Autodesk Inventor part; units mm, degrees
ref_plane "YZ Plane" through (0, 0, 0) normal (1, 0, 0) x (0, 1, 0)
ref_plane "XZ Plane" through (0, 0, 0) normal (0, 1, 0) x (-1, 0, 0)
ref_plane "XY Plane" through (0, 0, 0) normal (0, 0, 1) x (1, 0, 0)
sketch "Szkic1" plane through (0, 0, 0) normal (0, 1, 0) x (-1, 0, 0)
  line L0 (0, 0) -> (150, 0)
  line L1 (150, 0) -> (150, -5)
  line L2 (150, -5) -> (0, -5)
  line L3 (0, -5) -> (0, 0)
  dimension "d0" = 150
  dimension "d1" = 5
extrude "Wyciągnięcie proste1" add sketch "Szkic1" along normal blind 20
sketch "Szkic2" plane through (0, 0, -5) normal (0, 0, -1) x (-1, 0, 0)
  line L0 (0, 0) -> (0, 20)
  circle A0 centre (0, 10) radius 2.95
  line L1 (0, 20) -> (-2, 20)
  line L2 (0, 0) -> (-2, 0)
  arc A1 (-2, 20) -> (-2, 0) centre (9.1803, 10) ccw
  line L3 (0, 10) -> (150, 10)
  line L4 (150, 10) -> (138.5, 10)
  line L5 (138.5, 10) -> (170.9, 10)
  line L6 (150, 0) -> (150, 20)
  line L7 (138.5, 10) -> (170.9, 10) construction
  line L8 (138.5, 10) -> (170.9, 10)
  line L9 (170.9, 10) -> (170.9, 16.16)
  line L10 (170.9, 16.16) -> (138.5, 16.16)
  line L11 (138.5, 16.16) -> (138.5, 10)
  line L12 (138.5, 10) -> (170.9, 10)
  line L13 (170.9, 10) -> (170.9, 3.84)
  line L14 (170.9, 3.84) -> (138.5, 3.84)
  line L15 (138.5, 3.84) -> (138.5, 10)
  line L16 (0, 0) -> (150, 0)
  line L17 (0, 20) -> (150, 20)
  arc A2 (138.5, 0) -> (138.5, 20) centre (154.9429, 10) ccw
  point P0 (150, 3.84)
  point P1 (150, 16.16)
  point P2 (0, 7.05)
  point P3 (0, 12.95)
  dimension "d4" = 5.9
  dimension "d5" = 2
  dimension "d6" = 2
  dimension "d7" = 15
  dimension "d8" = 150
  dimension "d9" = 11.5
  dimension "d10" = 32.4
  dimension "d11" = 0
  dimension "d12" = 6.16
  dimension "d13" = 6.16
extrude "Wyciągnięcie proste2" add sketch "Szkic2" against normal blind 5 contours L2 A1 L1 L0 A0 | L16 L6 L14 L13 L9 L10 L17 A2
sketch "Szkic3" plane through (2, 20, -5) normal (0, 0, -1) x (-1, 0, 0)
  arc A0 (2, -7.05) -> (2, -12.95) centre (2, -10) ccw
  circle A1 centre (2, -10) radius 2.95
  line L0 (152, -16.16) -> (152, -3.84)
  line L1 (152, -16.16) -> (150.5, -16.16)
  line L2 (150.5, -16.16) -> (150.5, -3.84)
  line L3 (150.5, -3.84) -> (152, -3.84)
  line L4 (140.5, -16.16) -> (10.5, -16.16)
  line L5 (10.5, -16.16) -> (10.5, -3.84)
  line L6 (10.5, -3.84) -> (140.5, -3.84)
  line L7 (140.5, -3.84) -> (140.5, -16.16)
  line L8 (150.5, -16.16) -> (150.3, -16.16)
  line L9 (150.3, -16.16) -> (150.3, -3.84)
  line L10 (150.3, -3.84) -> (150.5, -3.84)
  line L11 (152, -16.16) -> (140.5, -16.16)
  line L12 (140.5, -16.16) -> (140.5, -3.84)
  line L13 (140.5, -3.84) -> (152, -3.84)
  line L14 (152, -3.84) -> (152, -16.16)
  point P0 (2, -20)
  dimension "d16" = 1.5
  dimension "d17" = 130
  dimension "d18" = 12.32
  dimension "d21" = 0.2
  dimension "d24" = 11.5
extrude "Wyciągnięcie proste3" cut sketch "Szkic3" against normal through all
sketch "Szkic5" plane through (2, 20, -5) normal (0, 0, -1) x (-1, 0, 0)
  circle A0 centre (2, -10) radius 2.95
  line L0 (2, -10) -> (152, -10)
  line L1 (2, -10) -> (152, -10) construction
  circle A1 centre (152, -10) radius 5.0551
  line L2 (152, -10) -> (145.8, -10)
  line L3 (145.8, -10) -> (145.8, -3.84)
  line L4 (10.5, -3.84) -> (172.9, -3.84)
  line L5 (145.8, -3.84) -> (140.8, -3.84)
  line L6 (140.8, -3.84) -> (140.8, -16.16)
  line L7 (172.9, -16.16) -> (10.5, -16.16)
  line L8 (145.8, -10) -> (145.8, -16.16)
  line L9 (145.8, -16.16) -> (140.8, -16.16)
  line L10 (10.5, -16.16) -> (10.5, -3.84)
  line L11 (10.5, -16.16) -> (44.3489, -3.84)
  line L12 (10.5, -16.16) -> (46.5213, -16.16) construction
  line L13 (44.3489, -3.84) -> (54.3489, -3.84)
  line L14 (10.5, -16.16) -> (20.5, -16.16)
  line L15 (20.5, -16.16) -> (54.3489, -3.84)
  line L16 (20.5, -16.16) -> (30.5, -16.16)
  line L17 (54.3489, -3.84) -> (64.3489, -3.84)
  line L18 (64.3489, -3.84) -> (30.5, -16.16)
  line L19 (44.3489, -3.84) -> (34.3489, -3.84)
  line L20 (10.5, -16.16) -> (0.5, -16.16)
  line L21 (0.5, -16.16) -> (34.3489, -3.84)
  line L22 (40.5, -16.16) -> (74.3489, -3.84)
  line L23 (50.5, -16.16) -> (84.3489, -3.84)
  line L24 (94.3489, -3.84) -> (60.5, -16.16)
  line L25 (30.5, -16.16) -> (64.3489, -3.84)
  line L26 (70.5, -16.16) -> (104.3489, -3.84)
  line L27 (80.5, -16.16) -> (114.3489, -3.84)
  line L28 (124.3489, -3.84) -> (90.5, -16.16)
  line L29 (60.5, -16.16) -> (94.3489, -3.84)
  line L30 (100.5, -16.16) -> (134.3489, -3.84)
  line L31 (110.5, -16.16) -> (144.3489, -3.84)
  line L32 (90.5, -16.16) -> (124.3489, -3.84)
  point P0 (2, -20)
  point P1 (10.5, -12.5203)
  point P2 (60.5, -16.16)
  point P3 (140.8, -5.1317)
  dimension "d25" = 150
  dimension "d26" = 0
  dimension "d27" = 6.2
  dimension "d28" = 5
  dimension "d29" = 20
  dimension "d30" = 10
  dimension "d31" = 10
  dimension "d32" = 10
  dimension "d33" = 10
  dimension "d34" = 10
  dimension "d35" = 10
  dimension "d36" = 10
  dimension "d37" = 10
  dimension "d38" = 10
  dimension "d39" = 10
  dimension "d40" = 10
  dimension "d41" = 10
  dimension "d42" = 10
  dimension "d43" = 10
  dimension "d44" = 10
  dimension "d45" = 10
  dimension "d46" = 10
  dimension "d47" = 10
  dimension "d48" = 10
  dimension "d49" = 10
  dimension "d52" = 10
  dimension "d53" = 10
extrude "Wyciągnięcie proste4" add sketch "Szkic5" against normal blind 5 contours L21 L4 L11 L0 | L0 L11 L10 L21 | L15 L4 L18 L0 | L0 L18 L7 L15 | L22 L4 L23 L0 | L0 L23 L7 L22 | L24 L4 L26 L0 | L0 L26 L7 L24 | L27 L4 L28 L0 | L0 L28 L7 L27 | L30 L4 L6 L31 L0 | L0 L31 L7 L30 | L6 L31 L4 L3 L0 | L0 L8 L7 L6 | L6 L4 L31
sketch "Szkic6" plane through (-138.5, 0, 0) normal (0, 0, 1) x (1, 0, 0)
  line L0 (-32.4, 16.16) -> (-32.4, 3.84)
  line L1 (-5.3, 3.84) -> (-32.4, 3.84)
  line L2 (-32.4, 16.16) -> (-5.3, 16.16)
  line L3 (-5.3, 16.16) -> (-5.3, 3.84)
  line L4 (-5.3, 3.84) -> (-32.4, 3.84)
  line L5 (-32.4, 3.84) -> (-32.4, 16.16)
  line L6 (-32.4, 16.16) -> (-33.4, 16.16)
  line L7 (-33.4, 16.16) -> (-33.4, 17.16)
  line L8 (-5.3, 3.84) -> (-5.3, 2.84)
  line L9 (-5.3, 2.84) -> (-4.3, 2.84)
  line L10 (-33.4, 17.16) -> (-4.3, 17.16)
  line L11 (-4.3, 17.16) -> (-4.3, 2.84)
  line L12 (-4.3, 2.84) -> (-33.4, 2.84)
  line L13 (-33.4, 2.84) -> (-33.4, 17.16)
  point P0 (138.5, 0)
  point P1 (-33.4, 16.16)
  dimension "d56" = 1
  dimension "d57" = 1
  dimension "d58" = 1
  dimension "d59" = 1
extrude "Wyciągnięcie proste5" add sketch "Szkic6" along normal blind 13 contours L6 L7 L10 L11 L9 L8 L3 L2 | L0 L1 L8 L12 L13 L6
sketch "Szkic7" plane through (-142.8, 2.84, 0) normal (1, 0, 0) x (0, 0, -1)
  line L0 (-13, 0) -> (-13, 14.32)
  line L1 (0, 17.16) -> (0, -2.84)
  line L2 (-13, 11.9333) -> (0, 11.9333)
  line L3 (0, 11.9333) -> (0, 3.1608)
  line L4 (0, 3.1608) -> (-13, 3.1608)
  line L5 (-13, 3.1608) -> (-13, 11.9333)
extrude "Wyciągnięcie proste6" cut sketch "Szkic7" against normal blind 8.75
sketch "Szkic8" plane through (-138.5, 0, 0) normal (0, 0, 1) x (1, 0, 0)
  circle A0 centre (138.5, 10) radius 2.95
  line L0 (138.5, 10) -> (-11.5, 10)
  circle A1 centre (-11.5, 10) radius 2.85
  line L1 (-14.35, 10) -> (-4.35, 10)
  line L2 (-4.35, 10) -> (-4.35, 16.6)
  line L3 (-4.35, 10) -> (2.25, 10) construction
  line L4 (-4.35, 10) -> (-4.35, 3.4)
  line L5 (-4.35, 16.6) -> (-32.35, 16.6)
  line L6 (-4.35, 16.6) -> (23.65, 16.6) construction
  line L7 (-32.35, 16.6) -> (-32.35, 3.4)
  line L8 (-32.35, 3.4) -> (-4.35, 3.4)
  point P0 (138.5, 0)
  dimension "d66" = 5.7
  dimension "d64" = 150
  dimension "d67" = 10
  dimension "d68" = 6.6
  dimension "d69" = 90
  dimension "d70" = 6.6
  dimension "d71" = 28
  dimension "d72" = 180
  dimension "d73" = 13.2
extrude "Wyciągnięcie proste7" cut sketch "Szkic8" along normal blind 22.75 and the other way blind 20.75 contours L4 L8 L7 L5 L2
sketch "Szkic10" plane through (-138.5, 0, 0) normal (0, 0, 1) x (1, 0, 0)
  line L0 (-4.3, 17.16) -> (-4.3, 14.7733)
  line L1 (-4.3, 14.7733) -> (-3.3, 14.7733)
  line L2 (-3.3, 14.7733) -> (-3.3, 17.16)
  line L3 (-3.3, 17.16) -> (-4.3, 17.16)
  line L4 (-4.3, 17.16) -> (-4.3, 14.7733)
  line L5 (-4.35, 14.7733) -> (-4.35, 6.0008)
  line L6 (-4.35, 6.0008) -> (-3.35, 6.0008)
  line L7 (-3.35, 6.0008) -> (-3.35, 2.8422)
  line L8 (-3.35, 2.8422) -> (-4.35, 2.8422)
  line L9 (-4.35, 2.8422) -> (-4.35, 6.0008)
  line L10 (-33.4, 17.16) -> (-4.3, 17.16)
  line L11 (-33.4, 17.16) -> (-3.3, 17.16)
  line L12 (-3.3, 17.16) -> (-3.3, 18.16)
  line L13 (-3.3, 18.16) -> (-33.4, 18.16)
  line L14 (-33.4, 18.16) -> (-33.4, 17.16)
  line L15 (-33.4, 2.8422) -> (-3.3, 2.8422)
  line L16 (-3.3, 2.8422) -> (-3.3, 1.8422)
  line L17 (-3.3, 1.8422) -> (-33.4, 1.8422)
  line L18 (-33.4, 1.8422) -> (-33.4, 2.8422)
  point P0 (138.5, 0)
  point P1 (-3.3, 17.16)
  point P2 (-3.35, 2.8422)
  dimension "d78" = 1
  dimension "d79" = 1
  dimension "d80" = 1
  dimension "d81" = 1
extrude "Wyciągnięcie proste8" add sketch "Szkic10" along normal blind 13
sketch "Szkic11" plane through (2, 20, -5) normal (0, 0, -1) x (-1, 0, 0)
  circle A0 centre (2, -10) radius 2.95
  line L0 (2, -10) -> (152, -10)
  line L1 (2, -10) -> (152, -10) construction
  circle A1 centre (152, -10) radius 2.4946
  point P0 (2, -20)
  dimension "d84" = 150
  dimension "d85" = 0
properties part number "arm_v3-1_backup"
The listing builds one solid part. Answer for the finished solid, in the listing's coordinates (mm). A direction names the side the tool comes from. Round coordinates to 2 decimals unless told otherwise and drop trailing zeros. Write each loop counter-clockwise with the first axis right and the second up, starting at its lowest first coordinate (ties: lowest second). Pieces come first, ordered by that corner, then holes. Notation, with made-up numbers: (-3, -35.75) -> (27, -35.75) arc R25 ccw to (27, -23.75) -> close; hole circle Ø3 at (13.5, 29). An arc over 180 degrees is marked (long way). Write item = value, one per line.
1) Section B-B on z = 10 is taken. Write down the section's boundary in (x, y), plus the area to 3 significant figures.
Check values:
outline = (-171.9, 1.84) -> (-141.8, 1.84) -> (-141.8, 2.84) -> (-141.85, 2.84) -> (-141.85, 6) -> (-142.85, 6) -> (-142.85, 3.4) -> (-170.85, 3.4) -> (-170.85, 3.84) -> (-170.9, 3.84) -> (-170.9, 16.16) -> (-170.85, 16.16) -> (-170.85, 16.6) -> (-142.85, 16.6) -> (-142.85, 14.77) -> (-141.8, 14.77) -> (-141.8, 18.16) -> (-171.9, 18.16) -> close
area = 112 mm²
2) Section A-A on x = 0 is taken. Write down the section's boundary in (y, z).
Check values:
outline = (0, -5) -> (7.05, -5) -> (7.05, 0) -> (0, 0) -> close; (12.95, -5) -> (20, -5) -> (20, 0) -> (12.95, 0) -> close
3) Section D-D on y = 10 is taken. Give the number of separate pieces and of enclosed holes in the cut face, plus the area to 3 significant figures.
Check values:
separate_pieces = 10
enclosed_holes = 0
area = 392 mm²
4) Given pin 1 (2.5 mm diameter, centred on x = -71.5, z = -2, fed in from +Y); pin 2 (10 mm diameter, centred on x = -149, z = 3, fed in from +Y); pin 3 (2.5 mm diameter, centred on y = 16.5, z = 5.5, fed in from +X), each flat-ended and moving along its own axis, determine where each tip first touches the part or whether it passes through.
Check values:
pin_1 = 20
pin_2 = 29.15
pin_3 = -141.8
5) For a pull along Y with two mould halves and no side action, classify faces 1 (the flat face through (-123.438, 9.277, -2.535)), 2 (the flat face through (-157, 18.16, 6)), 3 (the flat face through (-141.8, 16, 6)) as released by +Y, released by -Y, zero draft, split by the parting line, or undercut.
Check values:
face_1 = undercut
face_2 = released by +Y
face_3 = zero draft
6) Section C-C on x = -119 is taken. Write down the section's boundary in (y, z), plus the area to 3 significant figures.
Check values:
outline = (0, -5) -> (3.84, -5) -> (3.84, 0) -> (0, 0) -> close; (7.66, -5) -> (11.3, -5) -> (11.3, 0) -> (7.66, 0) -> close; (14.94, -5) -> (20, -5) -> (20, 0) -> (14.94, 0) -> close
area = 62.7 mm²
7) Which of the six approach directions +Z, -Z, +X, -X, +Y, -Y give full straight-line access (tool end or side, diameter ignored) to faces 4 (the flat face through (-85, 5, -5)), 5 (the flat face through (-95.188, 9.914, -2.535))?
Check values:
face_4 = -Z, +X, -X, +Y, -Y
face_5 = +Z, -Z
8) Straight lines are drawn through the part: line 1 along Y through (x, z) = (0, -2.95); line 2 along X through (y, z) = (5, 3.5); line 3 along Y through (x, z) = (-156, 11.5). For each, find the intervals that lie inside material, in ascending order. Write a range as [from, to].
Check values:
line_1 = [0, 7.05], [12.95, 20]
line_2 = [-171.9, -170.9], [-142.85, -141.85]
line_3 = [1.84, 3.4], [16.6, 18.16]
